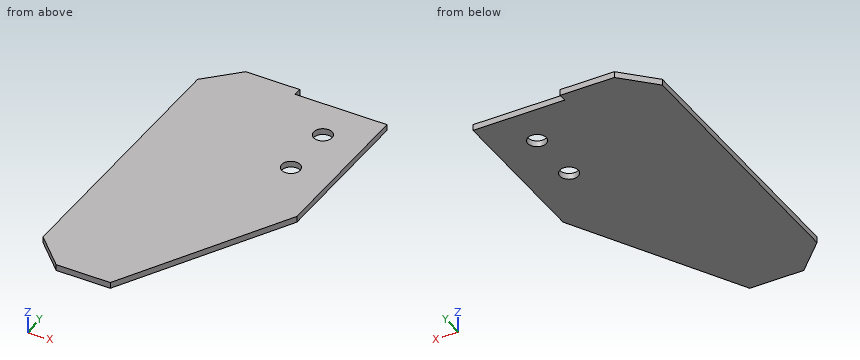
Autodesk Fusion 360 part; units mm, degrees
sketch "スケッチ1" plane through (0, 0, 0) normal (0, 0, 1) x (1, 0, 0)
  line L0 (-3.5, 163) -> (-86.5, 163)
  line L1 (-86.5, 163) -> (-86.5, -163)
  line L2 (-86.5, -163) -> (-3.5, -163)
  line L3 (86.5, 0) -> (86.5, 155)
  line L4 (82.2546, 155) -> (-86.5, -163) construction
  line L5 (-86.5, 163) -> (42.3924, -79.8839) construction
  line L6 (-3.5, 163) -> (-3.5, 155)
  line L7 (-3.5, 155) -> (86.5, 155)
  line L8 (-86.5, -163) -> (-3.5, -163) construction
  line L9 (86.5, 0) -> (-3.5, -163)
  dimension "d2" = 326
  dimension "d5" = 83
extrude "押し出し1" add sketch "スケッチ1" along normal blind 6
chamfer "面取り1" distance 30 angle 45 2 edges at (-86.5, -163, 3) (-86.5, 163, 3)
sketch "スケッチ2" plane through (0, 0, 6) normal (0, 0, 1) x (-1, 0, 0)
  line L0 (56.5, -163) -> (86.5, -133)
  line L1 (86.5, -133) -> (86.5, 133)
  line L2 (86.5, 133) -> (56.5, 163)
  line L3 (56.5, 163) -> (3.5, 163)
  line L4 (3.5, 163) -> (-86.5, 0)
  line L5 (-86.5, 0) -> (-86.5, -155)
  line L6 (-86.5, -155) -> (3.5, -155)
  line L7 (3.5, -155) -> (3.5, -163)
  line L8 (3.5, -163) -> (56.5, -163)
  line L9 (-86.5, -155) -> (-46.5, -155) construction
  line L10 (-46.5, -155) -> (-46.5, -115) construction
  line L11 (-46.5, -115) -> (-86.5, -115) construction
  line L12 (-86.5, -115) -> (-86.5, -155) construction
  line L13 (-46.5, -115) -> (-46.5, -60) construction
  point P0 (-46.5, -115)
  dimension "d10" = 40
  dimension "d11" = 40
  dimension "d12" = 55
hole "穴1" at (46.5, 115, 6) at (46.5, 60, 6) direction (0, 0, -1) diameter 18 end through all
equation "d5 = 30 mm + 53 mm"
CAD build for the part. Positions are in the model's coordinates, mm. Round coordinates to 2 decimals unless told otherwise and drop trailing zeros. Loops run counter-clockwise (first coordinate to the right, second up) from the corner with the lowest first, then second, coordinate; pieces in that order, holes last.
(1) Cut at C-C (x = 46.5). Give the cut face in (y, z), plus the area to 3 significant figures.
(2) Cut at A-A (y = 115). Give the cut face in (x, z).
(3) Wall check: line 1 along X through (y, z) = (115, 3.2); line 2 along Y through (x, z) = (46.5, 2.5); line 3 along X through (y, z) = (54.5, 2.2). Give the ranges that are in metal, low to high.
(4) Cut at D-D (y = -68). Give the cut face in (x, z), plus the area to 3 significant figures.
(5) Cut at B-B (z = 4.45). Give the cut face in (x, y), plus the area to 3 significant figures.
(6) Drop flat-ended pins along their axis: pin 1 (3 mm diameter, centred on y = -124, z = 1, fed in from +X); pin 2 (14.5 mm diameter, centred on x = 46.5, y = 115, fed in from -Z); pin 3 (3 mm diameter, centred on x = 35.5, z = 1.5, fed in from +Y). Give the stop position or say it passes through.
Findings below:
1. outline: (-72.44, 0) - (51, 0) - (51, 6) - (-72.44, 6) - close; (69, 0) - (106, 0) - (106, 6) - (69, 6) - close; (124, 0) - (155, 0) - (155, 6) - (124, 6) - close
1. area: 1,150 mm2
2. outline: (-86.5, 0) - (37.5, 0) - (37.5, 6) - (-86.5, 6) - close; (55.5, 0) - (86.5, 0) - (86.5, 6) - (55.5, 6) - close
3. line 1: x = -86.5 to 37.5, 55.5 to 86.5
3. line 2: y = -72.44 to 51, 69 to 106, 124 to 155
3. line 3: x = -86.5 to 39.38, 53.62 to 86.5
4. outline: (-86.5, 0) - (48.95, 0) - (48.95, 6) - (-86.5, 6) - close
4. area: 813 mm2
5. outline: (-86.5, -133) - (-56.5, -163) - (-3.5, -163) - (86.5, 0) - (86.5, 155) - (-3.5, 155) - (-3.5, 163) - (-56.5, 163) - (-86.5, 133) - close; hole circle Ø18 at (46.5, 60); hole circle Ø18 at (46.5, 115)
5. area: 46,900 mm2
6. pin 1: stops at x = 18.86
6. pin 2: passes through
6. pin 3: stops at y = 155
